Could you check a few things on this model? Use its own coordinates, in mm. Round coordinates to 2 decimals unless told otherwise and drop trailing zeros. Loops run counter-clockwise (first coordinate to the right, second up) from the corner with the lowest first, then second, coordinate; pieces in that order, holes last. Notation, with made-up numbers: (28.5, -13) -> (35.5, -13) arc R18 cw to (35.5, -4) -> close; hole circle Ø6 at (22.25, 63). An arc over 180 degrees is marked (long way). Write each question's results on one line, items separated by ' | '.
from build123d import *

# Parameters (mm, degrees)
SKETCH2_W           = 100
SKETCH2_H           = 140
BOSS_EXTRUDE1_DEPTH = 10
SKETCH3_R           = 5
MOUNTHOLE_DEPTH     = 5
SKETCH4_R           = 2
CUT_EXTRUDE2_DEPTH  = 101
SKETCH5_R           = 2
CUT_EXTRUDE3_DEPTH  = 101
SKETCH21_W          = 46
SKETCH21_H          = 55
SKETCH21_W_2        = 36
SKETCH21_H_2        = 26
CUT_EXTRUDE10_DEPTH = 11


with BuildPart() as part:
    # Sketch2 → Boss-Extrude1 (new body)
    with BuildSketch(Plane(origin=(0, 0, 0), x_dir=(1, 0, 0), z_dir=(0, 1, 0))):
        with Locations((50, 70)):
            Rectangle(SKETCH2_W, SKETCH2_H)
    extrude(amount=BOSS_EXTRUDE1_DEPTH)

    # Sketch3 → MountHole (cut)
    with BuildSketch(Plane(origin=(0, 10, 0), x_dir=(1, 0, 0), z_dir=(0, 1, 0))):
        with Locations((65, 100)):
            Circle(SKETCH3_R)
    extrude(amount=-MOUNTHOLE_DEPTH, mode=Mode.SUBTRACT)

    # Sketch4 → Cut-Extrude2 (cut, through all)
    with BuildSketch(Plane.ZY):
        with Locations((-8, 5)):
            Circle(SKETCH4_R)
    extrude(amount=-CUT_EXTRUDE2_DEPTH, mode=Mode.SUBTRACT)

    # Sketch5 → Cut-Extrude3 (cut, through all)
    with BuildSketch(Plane.ZY):
        with Locations((-132, 5)):
            Circle(SKETCH5_R)
    extrude(amount=-CUT_EXTRUDE3_DEPTH, mode=Mode.SUBTRACT)

    # Sketch21 → Cut-Extrude10 (cut, through all)
    with BuildSketch(Plane(origin=(0, 10, 0), x_dir=(1, 0, 0), z_dir=(0, 1, 0))):
        with Locations((30.5, 94)):
            Rectangle(SKETCH21_W, SKETCH21_H)
        with Locations((71.5, 43)):
            Rectangle(SKETCH21_W_2, SKETCH21_H_2)
    extrude(amount=-CUT_EXTRUDE10_DEPTH, mode=Mode.SUBTRACT)


solid = part.part
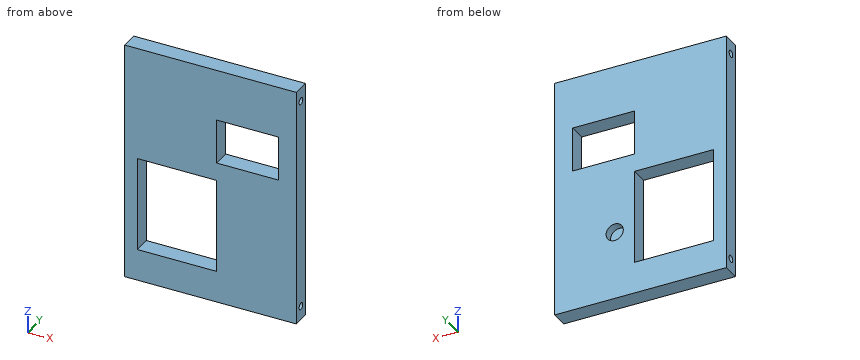
1) I want a section at D-D, the plane x = 94. Write out the boundary of the cut face in (y, z).
Model answer:
outline: (0, -140) -> (10, -140) -> (10, 0) -> (0, 0) -> close; hole circle Ø4 at (5, -132); hole circle Ø4 at (5, -8)
2) I want a section at C-C, the plane y = 8.5. Write out the boundary of the cut face in (x, z).
Model answer:
outline: (0, -140) -> (100, -140) -> (100, 0) -> (0, 0) -> close; hole (7.5, -121.5) -> (53.5, -121.5) -> (53.5, -66.5) -> (7.5, -66.5) -> close; hole (53.5, -56) -> (89.5, -56) -> (89.5, -30) -> (53.5, -30) -> close; hole circle Ø10 at (65, -100)
3) I'm going to push a flat-ended pin straight in: pin 1 (3 mm diameter, centred on y = 5, z = -8, fed in from +X). Where does the tip first touch, or does it pass through?
Model answer:
pin 1: passes through
4) I need wall thicknesses on line 1 (X direction, y = 6.5, z = -100); line 2 (Z direction, x = 65, y = 8.85); line 3 (Z direction, x = 10.5, y = 2.75). Which ranges of each line are inside material? Lowest first, please.
Model answer:
line 1: x = 0 to 7.5, 53.5 to 60, 70 to 100 | line 2: z = -140 to -105, -95 to -56, -30 to 0 | line 3: z = -140 to -121.5, -66.5 to 0
5) I want a section at B-B, the plane z = -88. Write out the boundary of the cut face in (x, y), plus the area to 3 significant figures.
Model answer:
outline: (0, 0) -> (7.5, 0) -> (7.5, 10) -> (0, 10) -> close; (53.5, 0) -> (100, 0) -> (100, 10) -> (53.5, 10) -> close | area: 540 mm2
6) I want a section at A-A, the plane x = 38. Write out the boundary of the cut face in (y, z), plus the area to 3 significant figures.
Model answer:
outline: (0, -140) -> (10, -140) -> (10, -121.5) -> (0, -121.5) -> close; (0, -66.5) -> (10, -66.5) -> (10, 0) -> (0, 0) -> close; hole circle Ø4 at (5, -132); hole circle Ø4 at (5, -8) | area: 825 mm2
